```python
from build123d import *

# Parameters (mm, degrees)
F0_W         = 101.0383963585
F0_H         = 60.3721439838
F1_DEPTH     = 31.0119315982
F3_SIZE2     = 2.54
F3_SIZE      = 5.08
F4_SIZE      = 12.7
F5_R         = 2.54
F6_T1_DEPTH  = 23.2584097937
F6_T3_DEPTH  = 23.2584097937
F6_T5_DEPTH  = 25.9319315982
F6_T10_DEPTH = 2.54
F6_T16_DEPTH = 2.54
F6_T22_DEPTH = 2.54
F6_T28_DEPTH = 2.54


# Not quite as in the source:
# - a fillet or chamfer that OpenCascade refuses, or shapes differently, is made with other operations: its cross-section is extruded or revolved along the edge and cut away or added


with BuildPart() as f1:
    # F0 (on Top) → F1 (new body)
    with BuildSketch(Plane.XY):
        Rectangle(F0_W, F0_H)
    extrude(amount=F1_DEPTH)

    # F3
    f3_edges = [f1.edges().sort_by_distance(p)[0] for p in [
        (0, -30.186072, 31.011932),
        (0, -30.186072, 0),
    ]]
    f3_side = f1.faces().sort_by_distance((0, -30.186072, 15.505966))[0]
    chamfer(f3_edges, length=F3_SIZE, length2=F3_SIZE2, reference=f3_side)

    # F4
    f4_edges = [f1.edges().sort_by_distance(p)[0] for p in [
        (50.519198, 30.186072, 15.505966),
        (-50.519198, 30.186072, 15.505966),
    ]]
    chamfer(f4_edges, length=F4_SIZE)

    # F5
    f5_edges = [f1.edges().sort_by_distance(p)[0] for p in [
        (50.519198, -30.186072, 15.505966),
        (50.519198, -28.916072, 28.471932),
        (50.519198, -5.08, 31.011932),
        (50.519198, -5.08, 0),
        (50.519198, -28.916072, 2.54),
        (-50.519198, -5.08, 31.011932),
        (-50.519198, -30.186072, 15.505966),
        (-50.519198, -28.916072, 28.471932),
        (-50.519198, -28.916072, 2.54),
        (-50.519198, -5.08, 0),
    ]]
    fillet(f5_edges, radius=F5_R)

    # F6: fillet of radius 2.54 on 6 edges, made by hand

    # F6_s2 → F6_t1 (cut)
    with BuildSketch(Plane(origin=(15.7726143179, -15.7726143179, 0), x_dir=(0, 0, 1), z_dir=(-0.7071067812, 0.7071067812, 0))):
        with BuildLine():
            ThreePointArc((28.4719315982, 48.0869876945), (30.2679828224, 47.3430389187), (31.0119315982, 45.5469876945))
            Line((31.0119315982, 45.5469876945), (31.0119315982, 48.0869876945))
            Line((31.0119315982, 48.0869876945), (28.4719315982, 48.0869876945))
        make_face()
        with BuildLine():
            ThreePointArc((2.54, 48.0869876945), (0.7439487758, 47.3430389187), (0, 45.5469876945))
            Line((0, 45.5469876945), (0, 48.0869876945))
            Line((0, 48.0869876945), (2.54, 48.0869876945))
        make_face()
    extrude(amount=F6_T1_DEPTH, mode=Mode.SUBTRACT)

    # F6_s4 → F6_t3 (cut)
    with BuildSketch(Plane(origin=(0.6735649669, 0.6735649669, 0), x_dir=(0, 0, 1), z_dir=(-0.7071067812, -0.7071067812, 0))):
        with BuildLine():
            ThreePointArc((31.0119315982, 45.5469876945), (30.2679828224, 47.3430389187), (28.4719315982, 48.0869876945))
            Line((28.4719315982, 48.0869876945), (31.0119315982, 48.0869876945))
            Line((31.0119315982, 48.0869876945), (31.0119315982, 45.5469876945))
        make_face()
        with BuildLine():
            ThreePointArc((0, 45.5469876945), (0.7439487758, 47.3430389187), (2.54, 48.0869876945))
            Line((2.54, 48.0869876945), (0, 48.0869876945))
            Line((0, 48.0869876945), (0, 45.5469876945))
        make_face()
    extrude(amount=F6_T3_DEPTH, mode=Mode.SUBTRACT)

    # F6_s6 → F6_t5 (cut)
    with BuildSketch(Plane.XY.offset(2.54)):
        with BuildLine():
            ThreePointArc((50.5191981792, 16.4339695435), (50.3258521918, 17.4059854617), (49.7752494035, 18.2300207677))
            Line((49.7752494035, 18.2300207677), (50.5191981792, 17.4860719919))
            Line((50.5191981792, 17.4860719919), (50.5191981792, 16.4339695435))
        make_face()
        with BuildLine():
            ThreePointArc((-49.7752494035, 18.2300207677), (-50.3258521918, 17.4059854617), (-50.5191981792, 16.4339695435))
            Line((-50.5191981792, 16.4339695435), (-50.5191981792, 17.4860719919))
            Line((-50.5191981792, 17.4860719919), (-49.7752494035, 18.2300207677))
        make_face()
    extrude(amount=F6_T5_DEPTH, mode=Mode.SUBTRACT)


with BuildPart() as f6_tool8:
    # F6_s9 → F6_t10 (new body)
    with BuildSketch(Plane.XY.offset(2.54)):
        Polygon((-47.9791981792, 16.4339695435), (-50.5191981792, 16.4339695435), (-50.5191981792, 17.4860719919), (-49.7752494035, 18.2300207677), align=None)
    extrude(amount=-F6_T10_DEPTH)

    # F6_s11 → F6_t12 (revolve, cut)
    with BuildSketch(Plane(origin=(-47.9791981792, 16.4339695435, 2.54), x_dir=(0.9238795325, -0.3826834324, 0), z_dir=(0.3826834324, 0.9238795325, 0))):
        with BuildLine():
            ThreePointArc((0, -2.54), (2.54, 0), (0, 2.54))
            Line((0, 2.54), (0, -2.54))
        make_face()
    revolve(axis=Axis((-47.9791981792, 16.4339695435, 2.54), (0, 0, -1)), mode=Mode.SUBTRACT)


with BuildPart() as f1_1:
    add(f1.part)

    # F6_t7: cut F6_tool8
    add(f6_tool8.part, mode=Mode.SUBTRACT)


with BuildPart() as f6_tool14:
    # F6_s15 → F6_t16 (new body)
    with BuildSketch(Plane.XY.offset(28.4719315982)):
        Polygon((-47.9791981792, 16.4339695435), (-50.5191981792, 16.4339695435), (-50.5191981792, 17.4860719919), (-49.7752494035, 18.2300207677), align=None)
    extrude(amount=F6_T16_DEPTH)

    # F6_s17 → F6_t18 (revolve, cut)
    with BuildSketch(Plane(origin=(-47.9791981792, 16.4339695435, 28.4719315982), x_dir=(0.9238795325, -0.3826834324, 0), z_dir=(-0.3826834324, -0.9238795325, 0))):
        with BuildLine():
            ThreePointArc((0, -2.54), (2.54, 0), (0, 2.54))
            Line((0, 2.54), (0, -2.54))
        make_face()
    revolve(axis=Axis((-47.9791981792, 16.4339695435, 28.4719315982), (0, 0, 1)), mode=Mode.SUBTRACT)


with BuildPart() as f1_2:
    add(f1_1.part)

    # F6_t13: cut F6_tool14
    add(f6_tool14.part, mode=Mode.SUBTRACT)


with BuildPart() as f6_tool20:
    # F6_s21 → F6_t22 (new body)
    with BuildSketch(Plane.XY.offset(2.54)):
        Polygon((47.9791981792, 16.4339695435), (50.5191981792, 16.4339695435), (50.5191981792, 17.4860719919), (49.7752494035, 18.2300207677), align=None)
    extrude(amount=-F6_T22_DEPTH)

    # F6_s23 → F6_t24 (revolve, cut)
    with BuildSketch(Plane(origin=(47.9791981792, 16.4339695435, 2.54), x_dir=(-0.9238795325, -0.3826834324, 0), z_dir=(0.3826834324, -0.9238795325, 0))):
        with BuildLine():
            ThreePointArc((0, -2.54), (2.54, 0), (0, 2.54))
            Line((0, 2.54), (0, -2.54))
        make_face()
    revolve(axis=Axis((47.9791981792, 16.4339695435, 2.54), (0, 0, -1)), mode=Mode.SUBTRACT)


with BuildPart() as f1_3:
    add(f1_2.part)

    # F6_t19: cut F6_tool20
    add(f6_tool20.part, mode=Mode.SUBTRACT)


with BuildPart() as f6_tool26:
    # F6_s27 → F6_t28 (new body)
    with BuildSketch(Plane.XY.offset(28.4719315982)):
        Polygon((47.9791981792, 16.4339695435), (50.5191981792, 16.4339695435), (50.5191981792, 17.4860719919), (49.7752494035, 18.2300207677), align=None)
    extrude(amount=F6_T28_DEPTH)

    # F6_s29 → F6_t30 (revolve, cut)
    with BuildSketch(Plane(origin=(47.9791981792, 16.4339695435, 28.4719315982), x_dir=(-0.9238795325, -0.3826834324, 0), z_dir=(-0.3826834324, 0.9238795325, 0))):
        with BuildLine():
            ThreePointArc((0, -2.54), (2.54, 0), (0, 2.54))
            Line((0, 2.54), (0, -2.54))
        make_face()
    revolve(axis=Axis((47.9791981792, 16.4339695435, 28.4719315982), (0, 0, 1)), mode=Mode.SUBTRACT)


with BuildPart() as f1_4:
    add(f1_3.part)

    # F6_t25: cut F6_tool26
    add(f6_tool26.part, mode=Mode.SUBTRACT)


solid = f1_4.part
```
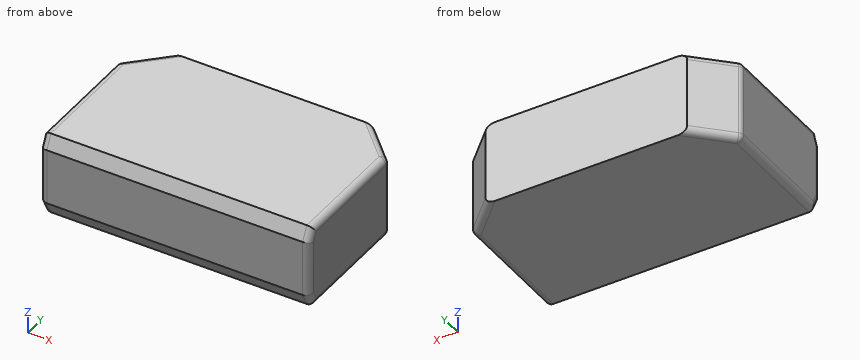
Here's how the part is built. I have some questions about the finished solid (model axes, mm). Give positions to 0.01 mm unless a question says otherwise; leave off trailing zeros. Loops run counter-clockwise (first coordinate to the right, second up) from the corner with the lowest first, then second, coordinate; pieces in that order, holes last. Notation, with made-up numbers: M 68,-9 L 107,-9 A12 ccw 107,8 Z; hole C 16,-15.5 d7. An arc over 180 degrees is marked long. Put each result on its own line as item: value. Start each with the question number.
(1) I want a section at A-A on z = 22. Please give me the cut outline in (x, y), then the cut area to 3 significant figures.
(2) I need wall thicknesses on line 1 along Y through (x, z) = (2, 2.5); line 2 along Y through (x, z) = (-23, 29); line 3 along X through (y, z) = (22.5, 15.5). Which ranges of each line are inside material? Lowest first, please. Write a range as [from, to].
(3) Will this pin go through, and if not, where does the flat tip stop? pin 1 Ø8 at (y, z) = (22.5, 5.5) entering from -X.
Answer block:
1. outline: M -50.52,-27.65 A2.54 ccw -47.98,-30.19 L 47.98,-30.19 A2.54 ccw 50.52,-27.65 L 50.52,16.43 A2.54 ccw 49.78,18.23 L 37.82,30.19 L -37.82,30.19 L -49.78,18.23 A2.54 ccw -50.52,16.43 Z
1. area: 5,940 mm^2
2. line 1: [-28.9, 30.19]
2. line 2: [-28.65, 30.19]
2. line 3: [-45.51, 45.51]
3. pin 1: x = -49.51
